Model file for the job. Use its own axes, mm. Give positions to 0.01 mm unless a question says otherwise; leave off trailing zeros. Write each loop counter-clockwise with the first axis right and the second up, starting at its lowest first coordinate (ties: lowest second). Pieces come first, ordered by that corner, then holes. Notation, with made-up numbers: M 31,26 L 45,26 A21 ccw 45,36 Z; hole C -18,82 d6. An arc over 180 degrees is marked long. Answer as a JSON object with one key per item and string values. Group by question number.
```python
from build123d import *

# Parameters (mm, degrees)
CROQUIS1_W              = 24.5
CROQUIS1_H              = 12.5
SALIENTE_EXTRUIR1_DEPTH = 3
CROQUIS2_R              = 0.5
CORTAR_EXTRUIR1_DEPTH   = 0.5
CROQUIS3_W              = 2
CROQUIS3_H              = 1.99806337
CROQUIS3_W_2            = 4
CROQUIS3_H_2            = 4
SALIENTE_EXTRUIR2_DEPTH = 0.8


with BuildPart() as part:
    # Croquis1 → Saliente-Extruir1 (new body)
    with BuildSketch(Plane(origin=(0, 0, 0), x_dir=(1, 0, 0), z_dir=(0, 1, 0))):
        Rectangle(CROQUIS1_W, CROQUIS1_H)
    extrude(amount=SALIENTE_EXTRUIR1_DEPTH)

    # Croquis2 → Cortar-Extruir1 (cut)
    with BuildSketch(Plane(origin=(0, 3, 0), x_dir=(1, 0, 0), z_dir=(0, 1, 0))):
        with Locations(Location((-7.654869521, -4.99629776, 0), (0, 0, 270))):
            Circle(CROQUIS2_R)
        with Locations(Location((-6.454869521, -4.99629776, 0), (0, 0, 270))):
            Circle(CROQUIS2_R)
        with Locations(Location((-5.254869521, -4.99629776, 0), (0, 0, 270))):
            Circle(CROQUIS2_R)
        with Locations(Location((-4.054869521, -4.99629776, 0), (0, 0, 270))):
            Circle(CROQUIS2_R)
    extrude(amount=-CORTAR_EXTRUIR1_DEPTH, mode=Mode.SUBTRACT)

    # Croquis3 → Saliente-Extruir2 (add)
    with BuildSketch(Plane(origin=(0, 3, 0), x_dir=(1, 0, 0), z_dir=(0, 1, 0))):
        with Locations((6.752485875, 1.575565117)):
            Rectangle(CROQUIS3_W, CROQUIS3_H)
        with Locations((-4.353841516, 2.457617945)):
            Rectangle(CROQUIS3_W_2, CROQUIS3_H_2)
        with Locations((6.752485875, 4.575565117)):
            Rectangle(CROQUIS3_W, CROQUIS3_H)
        with Locations((6.752485875, -1.424434883)):
            Rectangle(CROQUIS3_W, CROQUIS3_H)
    extrude(amount=SALIENTE_EXTRUIR2_DEPTH)


solid = part.part
```
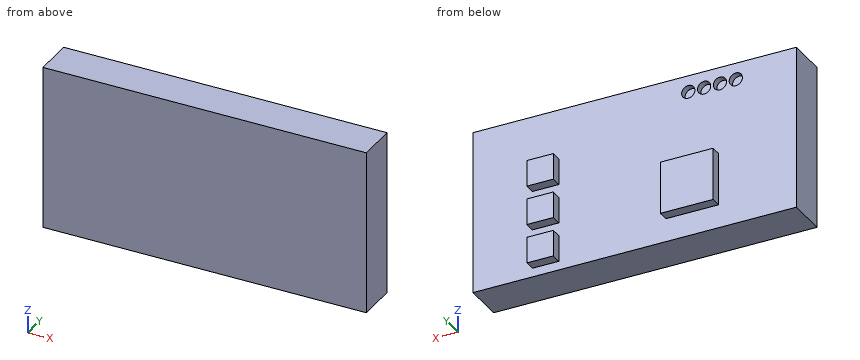
Q1. Drop flat-ended pins along their axis: P1, Ø0.9, axis at y = 3.5, z = -1.5, coming from the +X side; P2, Ø1.1, axis at x = -6.5, z = 5, coming from the +Y side; P3, Ø0.9, axis at y = 3.5, z = -2, coming from the -X side; P4, Ø2, axis at x = -10, z = -4.5, coming from the -Y side. Give the stop position or say it passes through.
Q2. Wall check: L1, parallel to Y at x = -9.75, z = -1.5; L2, parallel to X at y = 3.6, z = 1.75. Give the ranges that are in metal, low to high.
Q3. Slice it at A-A, the plane y = 3.5. Write the cut outline in (x, z), then the cut area to 3 significant figures.
Q4. Slice it at D-D, the plane z = -1.5. Write the cut outline in (x, y).
Q5. Slice it at C-C, the plane x = 1. Write the cut outline in (y, z).
Q6. Slice it at B-B, the plane z = 2. Write the cut outline in (x, y).
Solved:
{
 "1": {"P1": "stops at x = 7.75", "P2": "stops at y = 3", "P3": "stops at x = -6.35", "P4": "stops at y = 0"},
 "2": {"L1": "y = 0 to 3", "L2": "x = 5.75 to 7.75"},
 "3": {"outline": "M -6.35,-4.46 L -2.35,-4.46 L -2.35,-0.46 L -6.35,-0.46 Z; M 5.75,-5.57 L 7.75,-5.57 L 7.75,-3.58 L 5.75,-3.58 Z; M 5.75,-2.57 L 7.75,-2.57 L 7.75,-0.58 L 5.75,-0.58 Z; M 5.75,0.43 L 7.75,0.43 L 7.75,2.42 L 5.75,2.42 Z", "area": "28.0 mm²"},
 "4": {"outline": "M -12.25,0 L 12.25,0 L 12.25,3 L 7.75,3 L 7.75,3.8 L 5.75,3.8 L 5.75,3 L -2.35,3 L -2.35,3.8 L -6.35,3.8 L -6.35,3 L -12.25,3 Z"},
 "5": {"outline": "M 0,-6.25 L 3,-6.25 L 3,6.25 L 0,6.25 Z"},
 "6": {"outline": "M -12.25,0 L 12.25,0 L 12.25,3 L 7.75,3 L 7.75,3.8 L 5.75,3.8 L 5.75,3 L -12.25,3 Z"}
}
